Autodesk Inventor part; units mm, degrees
ref_plane "Work Plane1" through (0, 40, -50.485) normal (0, 0, -1) x (-1, 0, 0)
ref_plane "YZ Plane" through (0, 0, 0) normal (1, 0, 0) x (0, 1, 0)
ref_plane "XZ Plane" through (0, 0, 0) normal (0, 1, 0) x (-1, 0, 0)
sketch "Sketch1" plane through (0, 0, 0) normal (0, 1, 0) x (-1, 0, 0)
  circle A0 centre (0, 0) radius 67.5
  dimension "d0" = 135
extrude "body" add sketch "Sketch1" along normal blind 40
sketch "Sketch2" plane through (0, 40, 0) normal (0, 1, 0) x (1, 0, 0)
  circle A0 centre (0, 0) radius 67.5
  circle A1 centre (0, 0) radius 45.085
  dimension "d4" = 90.17
extrude "hole" cut sketch "Sketch2" against normal blind 101.6 contours A1
sketch "Sketch3" plane through (0, 40, 0) normal (0, 1, 0) x (1, 0, 0)
  circle A0 centre (0, 0) radius 45.085
  circle A1 centre (0, 0) radius 67.5
  circle A2 centre (0, 0) radius 50.485
  dimension "d9" = 5.4
extrude "flange" cut sketch "Sketch3" against normal blind 34 contours A1
sketch "Sketch4" plane through (0, 40, 0) normal (0, 1, 0) x (1, 0, 0)
  circle A0 centre (0, 0) radius 50.485
  circle A1 centre (0, 0) radius 45.085
  point P0 (0, 50.485)
ref_plane "Work Plane1" through (0, 40, -50.485) normal (0, 0, -1) x (-1, 0, 0)
sketch "Sketch5" plane through (0, 40, -50.485) normal (0, 0, -1) x (-1, 0, 0)
  circle A0 centre (0, -13) radius 2.54
  line L0 (50.485, 0) -> (-50.485, 0)
  point P0 (0, -40)
  dimension "d12" = 13
  dimension "d13" = 5.08
hole "sideHoleSE" at (0, 27, -50.485) direction (0, 0, 1) diameter 4.917 depth 17.1 tip angle 118
pattern_circular "sideHoleSW" count 2 over 120 about axis through (0, 40, 0) along (0, -1, 0) of "sideHoleSE"
pattern_circular "sideHoleN" count 2 over 120 about axis through (0, 40, 0) along (0, 1, 0) of "sideHoleSE"
sketch "Sketch8" plane through (0, 6, 0) normal (0, 1, 0) x (1, 0, 0)
  circle A0 centre (0, 0) radius 50.485
  circle A1 centre (0, 0) radius 67.5
  circle A2 centre (0, 57) radius 3.1903
  line L0 (0, 0) -> (49.3634, -28.5) construction
  line L1 (0, 0) -> (57, 0) construction
  circle A3 centre (49.3634, -28.5) radius 3.101
  line L2 (0, 0) -> (-51.9615, -30) construction
  line L3 (0, 0) -> (60, 0) construction
  circle A4 centre (-51.9615, -30) radius 3.5807
  dimension "d65" = 57
  dimension "d66" = 57
  dimension "d67" = 30
  dimension "d68" = 60
  dimension "d69" = 150
hole "Hole5" at (0, 6, -57) at (49.3634, 6, 28.5) at (-51.9615, 6, 30) direction (0, -1, 0) diameter 6.6 end through all
properties part number "2f1col" material "Aluminum 6061"
Geometry check sheet. Reference: the model listing, model coordinates, mm. A direction names the side the tool comes from. Give positions to 0.01 mm unless a question says otherwise; leave off trailing zeros. Order: outer loops, then holes, each group sorted by start corner. A loop starts at its lowest first (then second) coordinate and runs counter-clockwise, first axis right, second up. Notation, with made-up numbers: (57.25, 23) -> (106.25, 23) arc R15 cw to (106.25, 41) -> close; hole circle Ø1 at (17.5, -33.75). An arc over 180 degrees is marked (long way). Write each question's results on one line, items separated by ' | '. Start each with the question number.
(1) Sectioned sample at D-D (y = 27). Enter the section's corners in (x, z) (1 decimal).
(2) Sectioned sample at A-A (z = 0). Enter the section's corners in (x, y) (3 decimals), plus the area to 3 significant figures.
(3) Sectioned sample at C-C (z = 30). Enter the section's corners in (x, y).
(4) Gauge pin test, flat ends, axial feed: P1, Ø3, axis at x = 2.5, y = 6.5, coming from the +Z side; P2, Ø8, axis at y = 20, z = -42.5, coming from the -X side; P3, Ø10.5, axis at x = 0, z = -57, coming from the +Y side; P4, Ø5.5, axis at x = 49.36, z = 28.5, coming from the -Y side. Record the tip position at first contact, or that the pin passes through.
(5) Mould release check, pull along Z, two halves, no side actions. Record for faces 1 (the face through (-10.944, 23.238, 49.284)), 2 (the face through (40.85, 29.27, 24.67)), 3 (the face through (-41.79, 29.27, 23.04)), 4 (the face through (10, 6, 50)): pulls with the +Z half, pulls with the -Z half, needs draft (parallel to the pull), parting line crosses it, or undercut.
(6) Scan lines: line 1 (Z direction, x = 0, y = 3) (3 decimals); line 2 (X direction, y = 14, z = 0) (3 decimals). Record each from-to range of solid material in increasing order.
(7) Access from +Z, -Z, +X, -X, +Y, -Y to the whole of each face (thin tool, end or side, straight path). Record for faces 5 (the face through (1.5, 25.05, -47.71)), 6 (the face through (-9.774, 20.28, 44.013)).
(8) Sectioned sample at B-B (x = 0). Enter the section's corners in (y, z) (1 decimal).
Answer below:
1) outline: (-44.9, 23.1) arc R50.5 ccw to (-2.5, -50.4) -> (-2.5, -45) arc R45.1 cw to (-40.2, 20.4) -> close; (-42.4, 27.3) -> (-37.8, 24.6) arc R45.1 cw to (37.8, 24.6) -> (42.4, 27.3) arc R50.5 ccw to start; (2.5, -50.4) arc R50.5 ccw to (44.9, 23.1) -> (40.2, 20.4) arc R45.1 cw to (2.5, -45) -> close
2) outline: (-67.5, 0) -> (-45.085, 0) -> (-45.085, 40) -> (-50.485, 40) -> (-50.485, 6) -> (-67.5, 6) -> close; (45.085, 0) -> (67.5, 0) -> (67.5, 6) -> (50.485, 6) -> (50.485, 40) -> (45.085, 40) -> close | area: 636 mm2
3) outline: (-60.47, 0) -> (-55.26, 0) -> (-55.26, 6) -> (-60.47, 6) -> close; (-48.66, 0) -> (-33.65, 0) -> (-33.65, 40) -> (-40.6, 40) -> (-40.6, 6) -> (-48.66, 6) -> close; (33.65, 0) -> (46.42, 0) -> (46.42, 6) -> (40.6, 6) -> (40.6, 40) -> (33.65, 40) -> close; (52.3, 0) -> (60.47, 0) -> (60.47, 6) -> (52.3, 6) -> close
4) P1: z = 67.49 | P2: x = -32.66 | P3: y = 6 | P4: through
5) face 1: parting line crosses it | face 2: undercut | face 3: undercut | face 4: needs draft
6) line 1: -67.5 to -60.3, -53.7 to -45.085, 45.085 to 67.5 | line 2: -50.485 to -45.085, 45.085 to 50.485
7) face 5: -Z | face 6: +Y, -Y
8) outline: (0, -67.5) -> (6, -67.5) -> (6, -60.3) -> (0, -60.3) -> close; (0, -53.7) -> (6, -53.7) -> (6, -50.5) -> (24.5, -50.5) -> (24.5, -45.1) -> (0, -45.1) -> close; (0, 45.1) -> (40, 45.1) -> (40, 50.5) -> (6, 50.5) -> (6, 67.5) -> (0, 67.5) -> close; (29.5, -50.5) -> (40, -50.5) -> (40, -45.1) -> (29.5, -45.1) -> close
